from build123d import *

# Parameters (mm, degrees)
F2_SIZE  = 0.8128
F3_R     = 3.175
F4_DEPTH = 25.4


with BuildPart() as f1:
    # F0 (on Right) → F1 (revolve)
    with BuildSketch(Plane.YZ):
        Polygon((19.05, 34.925), (0, 34.925), (0, 31.877), (6.35, 31.877), (6.35, 8.4455), (12.2555, 8.4455), (19.05, 15.24), align=None)
    revolve(axis=Axis((0, 9.525, 0), (0, 1, 0)))

    # F2
    f2_edges = [f1.edges().sort_by_distance(p)[0] for p in [
        (0, 19.05, -34.925),
        (0, 0, -34.925),
        (0, 9.525, 34.925),
        (0, 0, -31.877),
    ]]
    chamfer(f2_edges, length=F2_SIZE)

    # F3 (on face) → F4 (cut)
    with BuildSketch(Plane(origin=(0, 19.05, 0), x_dir=(-1, 0, 0), z_dir=(0, 1, 0))):
        with Locations((0, 20.6375)):
            Circle(F3_R)
    extrude(amount=-F4_DEPTH, mode=Mode.SUBTRACT)


solid = f1.part
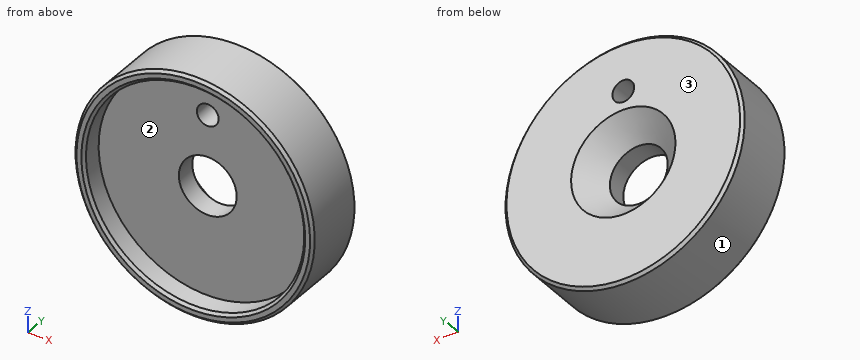
Design review of the part built by this model. Coordinates are the model's own, in mm. Face numbers are marked on the shaded views. Give positions to 0.01 mm unless a question says otherwise; leave off trailing zeros. Loops run counter-clockwise (first coordinate to the right, second up) from the corner with the lowest first, then second, coordinate; pieces in that order, holes last. Notation, with made-up numbers: (-35, 76) -> (-13, 76) arc R14 cw to (-13, 90) -> close; hole circle Ø2 at (3.5, 9). An arc over 180 degrees is marked (long way). One line per question, with ' | ' between items. Start each with the question number.
(1) We need section C-C (y = 3.75). State the section outline as (x, z) points (3 decimals).
(2) We need section B-B (x = 0). State how many separate pieces and enclosed holes the cut face has, and give its area (3 significant figures).
(3) For line 1 (X direction, y = 3.4, z = 0) (3 decimals); line 2 (X direction, y = 10.45, z = 0) (1 decimal); line 3 (Y direction, x = 14.5, z = 24.5), list the stretches that pass through material, from the lowest coordinate up.
(4) Draft analysis for pull direction Z (two halves, no side actions). For the marked faces 1, 2 and 3, state which applies: +Z half, -Z half, draft (parallel to the pull), parting line (faces both ways), or undercut.
(5) Insertion check: P1, Ø1.5, axis at x = -8.5, z = 3.5, coming from the +Y side; P2, Ø3, axis at x = -18, y = 11, coming from the +Z side; P3, Ø8, axis at y = 4, z = -21, coming from the -X side. Each pin has a flat end and moves straight along its axis. Give the tip position at first contact, or say it passes through.
The answers:
1) outline: circle Ø69.85 at (0, 0); hole circle Ø63.754 at (0, 0)
2) separate pieces: 3 | enclosed holes: 0 | area: 582 mm^2
3) line 1: x = -34.925 to -31.877, 31.877 to 34.925 | line 2: x = -34.9 to -8.4, 8.4 to 34.9 | line 3: y = 6.35 to 19.05
4) face 1: parting line | face 2: undercut | face 3: draft
5) P1: stops at y = 13.75 | P2: stops at z = 30.78 | P3: stops at x = -30.51
